Input: dimensioned drawing with shaded views. Units: mm. Origin: part minimum x, y, z. A direction names the side the tool comes from. Round coordinates to 2 decimals unless told otherwise and drop trailing zeros. Order: outer loops, then holes, each group sorted by start corner. A loop starts at its lowest first (then second) coordinate and runs counter-clockwise, first axis right, second up. Notation, with made-up numbers: (41.5, 21.25) - (57.5, 21.25) arc R29 cw to (57.5, 42.25) - close; hole circle Ø11 at (77, 87.25). An arc over 180 degrees is marked (long way). Return JSON: item names as keys, results as strings. Group by question number.
1) Ray query, line 1 (X direction, y = 5.5, z = 15); line 2 (Y direction, x = 51, z = 29.25); line 3 (Y direction, x = 0.6, z = 15). Return the intervals inside material, ascending. Write a range as from..to.
2) Access query for the marked faces 1 and 2. Directions: +Z, -Z, +X, -X, +Y, -Y. A direction counts if a zero-diameter tool reaches every point of the face in a straight line with its end or side. Return the directions, or none.
3) Section D-D, the plane y = 16.25. Return loops of the section in (x, z).
4) Mould query, pull axis X, two halves, no side actions, for the marked faces 3, 4 and 5. Classes: pulls with the +X half, pulls with the -X half, needs draft (parallel to the pull), parting line crosses it, or undercut.
5) Contact query for flat-ended pins moving along their axis: P1, Ø4.5, axis at x = 11, y = 10, coming from the -Z side; P2, Ø4, axis at x = 14.5, z = 24, coming from the +Y side. Output: stop coordinate, or through.
6) Section B-B, the plane x = 51. Return loops of the section in (y, z).
7) Section A-A, the plane z = 23.5. Return loops of the section in (x, y), plus the area to 3 significant figures.
8) Section C-C, the plane z = 15. Return loops of the section in (x, y), plus the area to 3 significant figures.
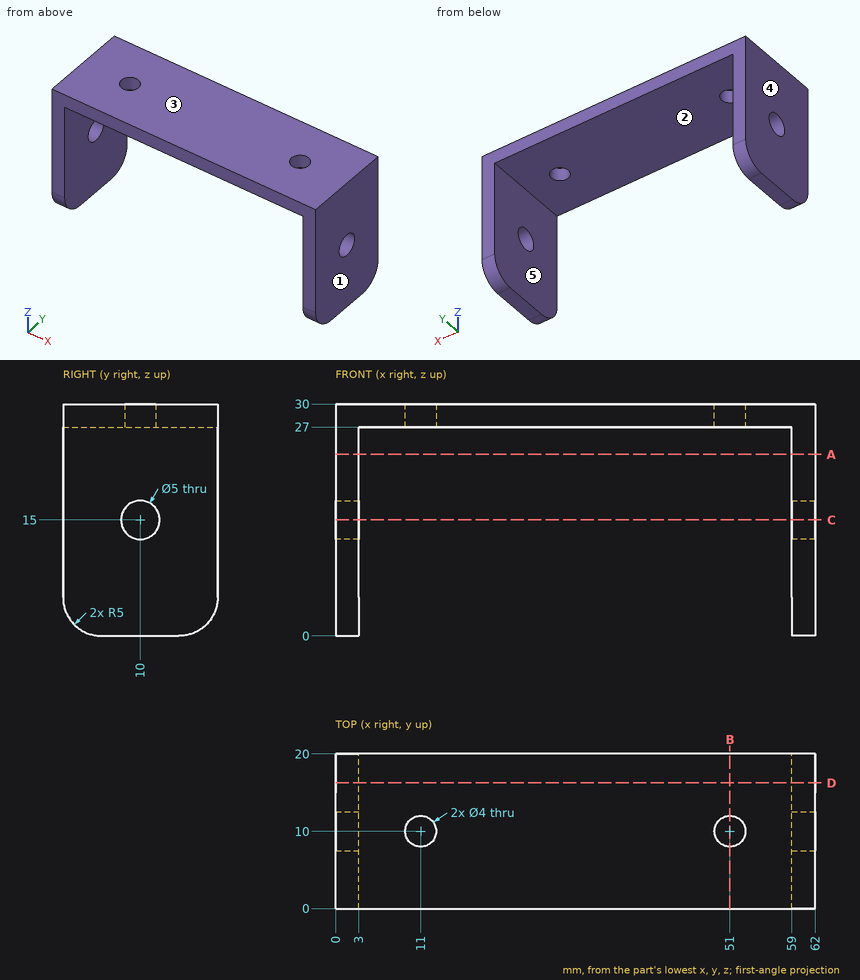
Geometry check:
{
 "1": {"line 1": "0..3, 59..62", "line 2": "0..8, 12..20", "line 3": "0..7.5, 12.5..20"},
 "2": {"face 1": "+Z, -Z, +X, +Y, -Y", "face 2": "-Z, +Y, -Y"},
 "3": {"outline": "(0, 0.16) - (3, 0.16) - (3, 27) - (59, 27) - (59, 0.16) - (62, 0.16) - (62, 30) - (0, 30) - close"},
 "4": {"face 3": "needs draft", "face 4": "pulls with the -X half", "face 5": "undercut"},
 "5": {"P1": "z = 27", "P2": "through"},
 "6": {"outline": "(0, 27) - (8, 27) - (8, 30) - (0, 30) - close; (12, 27) - (20, 27) - (20, 30) - (12, 30) - close"},
 "7": {"outline": "(0, 0) - (3, 0) - (3, 20) - (0, 20) - close; (59, 0) - (62, 0) - (62, 20) - (59, 20) - close", "area": "120 mm2"},
 "8": {"outline": "(0, 0) - (3, 0) - (3, 7.5) - (0, 7.5) - close; (0, 12.5) - (3, 12.5) - (3, 20) - (0, 20) - close; (59, 0) - (62, 0) - (62, 7.5) - (59, 7.5) - close; (59, 12.5) - (62, 12.5) - (62, 20) - (59, 20) - close", "area": "90.0 mm2"}
}
